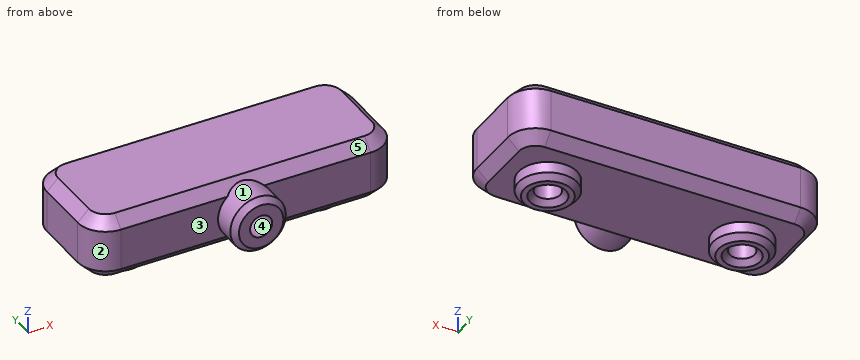
from build123d import *

# Parameters (mm, degrees)
SKETCH1_W                = 139.7
SKETCH1_H                = 50.8
SKETCH1_R                = 5.715
BOSS_EXTRUDE1_DEPTH      = 22.86
BOSS_EXTRUDE2_START      = 22.86
BOSS_EXTRUDE2_OUTLINE_W  = 139.7
BOSS_EXTRUDE2_OUTLINE_H  = 50.8
BOSS_EXTRUDE2_DEPTH      = 6.35
EXTRUDE_THIN1_START      = -7.62
SKETCH1_4_R              = 13.335
SKETCH1_4_R_2            = 5.715
EXTRUDE_THIN1_DEPTH      = 7.62
FILLET1_R                = 12.7
CHAMFER1_SIZE            = 5.08
CHAMFER3_SIZE            = 2.54
BOSS_EXTRUDE3_DEPTH      = 12.7
BOSS_EXTRUDE3_DEPTH_BACK = 12.7
SKETCH2_R                = 12.7
SKETCH2_R_2              = 5.08
CUT_EXTRUDE1_START       = -26.67
SKETCH2_2_R              = 5.08
CUT_EXTRUDE1_DEPTH       = 26.67
CHAMFER2_SIZE            = 2.54


# Read off the part's stored shape, not the designer's step: Boss-Extrude2
with BuildPart() as part:
    # Sketch1 → Boss-Extrude1 (new body)
    with BuildSketch(Plane.XY):
        Rectangle(SKETCH1_W, SKETCH1_H)
        with Locations((44.45, 0)):
            Circle(SKETCH1_R, mode=Mode.SUBTRACT)
        with Locations((-44.45, 0)):
            Circle(SKETCH1_R, mode=Mode.SUBTRACT)
    extrude(amount=BOSS_EXTRUDE1_DEPTH)

    # Boss-Extrude2 outline → Boss-Extrude2 (add)
    with BuildSketch(Plane.XY.offset(BOSS_EXTRUDE2_START)):
        Rectangle(BOSS_EXTRUDE2_OUTLINE_W, BOSS_EXTRUDE2_OUTLINE_H)
    extrude(amount=BOSS_EXTRUDE2_DEPTH)

    # Sketch1<4> → Extrude-Thin1 (add)
    # profile 1 of 2: a face of its own
    with BuildSketch(Plane.XY.offset(EXTRUDE_THIN1_START)):
        with Locations((44.45, 0)):
            Circle(SKETCH1_4_R)
        with Locations((44.45, 0)):
            Circle(SKETCH1_4_R_2, mode=Mode.SUBTRACT)
    # profile 2 of 2: a face of its own
    with BuildSketch(Plane.XY.offset(EXTRUDE_THIN1_START)):
        with Locations((-44.45, 0)):
            Circle(SKETCH1_4_R)
        with Locations((-44.45, 0)):
            Circle(SKETCH1_4_R_2, mode=Mode.SUBTRACT)
    extrude(amount=EXTRUDE_THIN1_DEPTH)

    # Fillet1
    fillet1_edges = [part.edges().sort_by_distance(p)[0] for p in [
        (-69.85, 25.4, 14.605),
        (69.85, 25.4, 14.605),
        (69.85, -25.4, 14.605),
        (-69.85, -25.4, 14.605),
    ]]
    fillet(fillet1_edges, radius=FILLET1_R)

    # Chamfer1
    chamfer1_edges = [part.edges().sort_by_distance(p)[0] for p in [
        (0, -25.4, 0),
        (0, -25.4, 29.21),
        (-69.85, 0, 0),
        (0, 25.4, 0),
        (69.85, 0, 0),
        (-66.130256121, 21.680256121, 0),
        (66.130256121, 21.680256121, 0),
        (66.130256121, -21.680256121, 0),
        (-66.130256121, -21.680256121, 0),
        (-69.85, 0, 29.21),
        (69.85, 0, 29.21),
        (0, 25.4, 29.21),
        (-66.130256121, 21.680256121, 29.21),
        (66.130256121, 21.680256121, 29.21),
        (66.130256121, -21.680256121, 29.21),
        (-66.130256121, -21.680256121, 29.21),
    ]]
    chamfer(chamfer1_edges, length=CHAMFER1_SIZE)

    # Chamfer3
    chamfer3_edges = [part.edges().sort_by_distance(p)[0] for p in [
        (31.115, 0, -7.62),
        (38.735, 0, -7.62),
        (-57.785, 0, -7.62),
        (-50.165, 0, -7.62),
    ]]
    chamfer(chamfer3_edges, length=CHAMFER3_SIZE)

    # Sketch2 → Boss-Extrude3 (add, two sides: drawn at the far end of the back side and taken through both)
    with BuildSketch(Plane.XZ.offset(25.4).offset(-BOSS_EXTRUDE3_DEPTH_BACK)):
        with Locations((0, 14.605)):
            Circle(SKETCH2_R)
        with Locations((0, 14.605)):
            Circle(SKETCH2_R_2, mode=Mode.SUBTRACT)
    extrude(amount=BOSS_EXTRUDE3_DEPTH + BOSS_EXTRUDE3_DEPTH_BACK)

    # Sketch2<2> → Cut-Extrude1 (cut)
    with BuildSketch(Plane.XZ.offset(25.4).offset(CUT_EXTRUDE1_START)):
        with Locations((0, 14.605)):
            Circle(SKETCH2_2_R)
    extrude(amount=CUT_EXTRUDE1_DEPTH, mode=Mode.SUBTRACT)

    # Chamfer2
    chamfer2_edges = [part.edges().sort_by_distance(p)[0] for p in [
        (-12.7, -38.1, 14.605),
    ]]
    chamfer(chamfer2_edges, length=CHAMFER2_SIZE)


solid = part.part
Verification items for the finished model (mm, model axes). Face numbers are marked on the shaded views. A direction names the side the tool comes from. Coordinates: 2 decimals unless noted, no trailing zeros. Order: outer loops, then holes, each group sorted by start corner. A loop starts at its lowest first (then second) coordinate and runs counter-clockwise, first axis right, second up. Notation, with made-up numbers: (86.5, 40.25) -> (110.5, 40.25) arc R17 cw to (110.5, 66.25) -> close; hole circle Ø10 at (12, 66.25). An arc over 180 degrees is marked (long way). Put each result on its own line as item: value. Start each with the question number.
1. Cross-section at B-B, the plane z = -1.5. Record the boundary of the cut face in (x, y) (3 decimals).
2. Mould release check, pull along Z, two halves, no side actions. Record for the marked faces 3, 4 and 5: released by +Z, released by -Z, zero draft, split by the parting line, or undercut.
3. Material ranges on L1, parallel to Y at x = -44.45, z = 9 (3 decimals); L2, parallel to X at y = -2, z = 11.5; L3, parallel to Z at x = 0, y = -18.5 (3 decimals), recorded low to high. Write a range as [from, to].
4. Go/stop test with flat-tipped pins: pin 1 Ø10 at (x, y) = (30.5, 14) entering from -Z; pin 2 Ø9 at (x, y) = (42.5, -2) entering from -Z; pin 3 Ø9.5 at (x, z) = (-39.5, 11.5) entering from -Y. Record where each tip stops, or that it passes through.
5. Access from +Z, -Z, +X, -X, +Y, -Y to the whole of each face (thin tool, end or side, straight path). Record for the marked faces 1 and 2.
6. Cross-section at A-A, the plane x = 0. Record the boundary of the cut face in (y, z) (3 decimals).
7. Cross-section at D-D, the plane x = -17.5. Record the boundary of the cut face in (y, z).
Computed:
1. outline: circle Ø26.67 at (-44.45, 0); circle Ø26.67 at (44.45, 0); hole circle Ø11.43 at (-44.45, 0); hole circle Ø11.43 at (44.45, 0)
2. face 3: zero draft
2. face 4: undercut
2. face 5: released by +Z
3. L1: [-25.4, -5.715], [5.715, 25.4]
3. L2: [-69.85, -49.8], [-39.1, -4.02], [4.02, 39.1], [49.8, 69.85]
3. L3: [0, 9.525], [19.685, 29.21]
4. pin 1: z = 0
4. pin 2: z = -6.66
4. pin 3: y = -25.4
5. face 1: -Y
5. face 2: +Z, -Z, -X, -Y
6. outline: (-38.1, 4.445) -> (-35.56, 1.905) -> (-22.225, 1.905) -> (-20.32, 0) -> (20.32, 0) -> (25.4, 5.08) -> (25.4, 24.13) -> (20.32, 29.21) -> (-20.32, 29.21) -> (-22.225, 27.305) -> (-35.56, 27.305) -> (-38.1, 24.765) -> (-38.1, 19.685) -> (1.27, 19.685) -> (1.27, 9.525) -> (-38.1, 9.525) -> close
7. outline: (-25.4, 5.08) -> (-20.32, 0) -> (20.32, 0) -> (25.4, 5.08) -> (25.4, 24.13) -> (20.32, 29.21) -> (-20.32, 29.21) -> (-25.4, 24.13) -> close
